Read the model definition and answer for the solid it produces. Units are mm, in the model's axes. Coordinates: 2 decimals unless noted, no trailing zeros. Order: outer loops, then holes, each group sorted by start corner. A loop starts at its lowest first (then second) coordinate and runs counter-clockwise, first axis right, second up.
```python
from build123d import *

# Parameters (mm, degrees)
F0_R     = 19.05
F1_DEPTH = 38.1
F3_DEPTH = 25.4
F5_DEPTH = 25.4
F6_R     = 9.525
F7_DEPTH = 138.43


with BuildPart() as f1:
    # F0 (on Front) → F1 (new body, symmetric)
    with BuildSketch(Plane.XZ):
        Circle(F0_R)
    extrude(amount=F1_DEPTH, both=True)

    # F2 (on face) → F3 (join)
    with BuildSketch(Plane(origin=(0, 38.1, 0), x_dir=(-1, 0, 0), z_dir=(0, 1, 0))):
        with BuildLine():
            ThreePointArc((-19.05, 0), (0, 19.05), (19.05, 0))
            Line((19.05, 0), (19.05, 76.2))
            Line((19.05, 76.2), (-19.05, 76.2))
            Line((-19.05, 76.2), (-19.05, 0))
        make_face()
        with BuildLine():
            Line((-19.05, 76.2), (19.05, 76.2))
            ThreePointArc((19.05, 76.2), (0, 95.25), (-19.05, 76.2))
        make_face()
        with BuildLine():
            ThreePointArc((-19.05, 0), (0, -19.05), (19.05, 0))
            ThreePointArc((19.05, 0), (0, 19.05), (-19.05, 0))
        make_face()
    extrude(amount=F3_DEPTH)

    # F4 (on face) → F5 (join)
    with BuildSketch(Plane.XZ.offset(38.1)):
        with BuildLine():
            Line((-19.05, 76.2), (19.05, 76.2))
            ThreePointArc((19.05, 76.2), (0, 95.25), (-19.05, 76.2))
        make_face()
        with BuildLine():
            ThreePointArc((-19.05, 0), (0, 19.05), (19.05, 0))
            Line((19.05, 0), (19.05, 76.2))
            Line((19.05, 76.2), (-19.05, 76.2))
            Line((-19.05, 76.2), (-19.05, 0))
        make_face()
        with BuildLine():
            ThreePointArc((-19.05, 0), (0, -19.05), (19.05, 0))
            ThreePointArc((19.05, 0), (0, 19.05), (-19.05, 0))
        make_face()
    extrude(amount=F5_DEPTH)

    # F6 (on face) → F7 (cut)
    with BuildSketch(Plane.XZ.offset(63.5)):
        with Locations((0, 76.2)):
            Circle(F6_R)
        Circle(F6_R)
    extrude(amount=-F7_DEPTH, mode=Mode.SUBTRACT)


solid = f1.part
```
1) Determine the mould class of faces 1 (the cylindrical face through (-4.13, 0.889, -18.597)), 2 (the cylindrical face through (4.4, -50.98, 67.75)), 3 (the flat face through (19.05, -51, 38)) for opening direction Z: pulls with the +Z half, pulls with the -Z half, needs draft (parallel to the pull), parting line crosses it, or undercut.
A:
face 1: parting line crosses it
face 2: undercut
face 3: needs draft
2) A cutting plane is placed at A-A, the plane x = 0. Determine the outline of the cut face in (y, z) (3 decimals).
A:
outline: (-63.5, -19.05) - (63.5, -19.05) - (63.5, -9.525) - (-63.5, -9.525) - close; (-63.5, 9.525) - (63.5, 9.525) - (63.5, 66.675) - (38.1, 66.675) - (38.1, 19.05) - (-38.1, 19.05) - (-38.1, 66.675) - (-63.5, 66.675) - close; (-63.5, 85.725) - (-38.1, 85.725) - (-38.1, 95.25) - (-63.5, 95.25) - close; (38.1, 85.725) - (63.5, 85.725) - (63.5, 95.25) - (38.1, 95.25) - close
3) A cutting plane is placed at C-C, the plane y = -52. Determine the outline of the cut face in (x, z) (3 decimals), and give its area (3 significant figures).
A:
outline: (-19.05, 0) arc R19.05 ccw to (19.05, 0) - (19.05, 76.2) arc R19.05 ccw to (-19.05, 76.2) - close; hole circle Ø19.05 at (0, 0); hole circle Ø19.05 at (0, 76.2)
area: 3,470 mm2
4) Straight lines are drawn through the part: line 1 (Z direction, x = 0, y = 55.5) (3 decimals); line 2 (Z direction, x = 2, y = 45); line 3 (Z direction, x = 0, y = -2) (3 decimals). For each, find the intervals that lie inside material, in ascending order.
A:
line 1: z = -19.05 to -9.525, 9.525 to 66.675, 85.725 to 95.25
line 2: z = -18.94 to -9.31, 9.31 to 66.89, 85.51 to 95.14
line 3: z = -19.05 to -9.525, 9.525 to 19.05
5) A cutting plane is placed at D-D, the plane z = 71. Determine the outline of the cut face in (x, y), and give its area (3 significant figures).
A:
outline: (-19.05, -63.5) - (-7.98, -63.5) - (-7.98, -38.1) - (-19.05, -38.1) - close; (-19.05, 38.1) - (-7.98, 38.1) - (-7.98, 63.5) - (-19.05, 63.5) - close; (7.98, -63.5) - (19.05, -63.5) - (19.05, -38.1) - (7.98, -38.1) - close; (7.98, 38.1) - (19.05, 38.1) - (19.05, 63.5) - (7.98, 63.5) - close
area: 1,120 mm2
6) A cutting plane is placed at B-B, the plane z = 22. Determine the outline of the cut face in (x, y).
A:
outline: (-19.05, -63.5) - (19.05, -63.5) - (19.05, -38.1) - (-19.05, -38.1) - close; (-19.05, 38.1) - (19.05, 38.1) - (19.05, 63.5) - (-19.05, 63.5) - close
7) Flat-ended cylindrical pins translate along their axes: pin 1 Ø6 at (y, z) = (-36.5, -6.5) entering from -X; pin 2 Ø4 at (x, z) = (9, 77) entering from +Y; pin 3 Ø2 at (x, y) = (-13, 31.5) entering from -Z. Find the tip coordinate at first contact, or state that the pin passes through.
A:
pin 1: stops at x = -18.73
pin 2: stops at y = 63.5
pin 3: stops at z = -14.8
